Read the model definition and answer for the solid it produces. Units are mm, in the model's axes. Coordinates: 2 decimals unless noted, no trailing zeros. Loops run counter-clockwise (first coordinate to the right, second up) from the corner with the lowest first, then second, coordinate; pieces in that order, holes last. Notation, with made-up numbers: (73.25, -35) -> (118.25, -35) arc R6 ccw to (118.25, -25) -> close; hole circle Ø6 at (-28.75, -19). An arc over 180 degrees is marked (long way). Answer as a JSON object with one key per item and string values. Group by question number.
1) Section C-C, the plane z = 4.25 is taken. Give the vertices of the cut face in (x, y).
2) Consider probe 1 along Y at (x, z) = (0, 18.75); probe 2 along X at (y, z) = (3.5, 1.5); probe 3 along Y at (x, z) = (-1, 21.5). Determine where each line is inside the solid, lowest interval first. Write a range as [from, to].
3) Flat-ended cylindrical pins translate along their axes: P1, Ø1.5, axis at x = 1, z = 9.5, coming from the -Y side; P2, Ø1.5, axis at x = -4, z = 20.5, coming from the -Y side; P3, Ø1, axis at y = -2, z = 4.5, coming from the +X side. Find the tip coordinate at first contact, or state that the pin passes through.
4) Section A-A, the plane x = 0 is taken. Give the vertices of the cut face in (y, z), plus the area to 3 significant figures.
5) Determine the mould class of faces 1 (the face through (-0.867, -3.905, 12.161)), 2 (the face through (-7.493, -0.33, 11.839)), 3 (the face through (5, 0, 0)) for opening direction X: released by +X, released by -X, zero draft, split by the parting line, or undercut.
Autodesk Inventor part; units mm, degrees
ref_plane "YZ Plane" through (0, 0, 0) normal (1, 0, 0) x (0, 1, 0)
ref_plane "XZ Plane" through (0, 0, 0) normal (0, 1, 0) x (-1, 0, 0)
ref_plane "XY Plane" through (0, 0, 0) normal (0, 0, 1) x (1, 0, 0)
sketch "Sketch1" plane through (0, 0, 0) normal (0, 0, 1) x (1, 0, 0)
  circle A0 centre (0, 0) radius 7.5
  dimension "d0" = 15
extrude "Extrusion1" add sketch "Sketch1" along normal blind 24
sketch "Sketch2" plane through (0, 0, 24) normal (0, 0, 1) x (1, 0, 0)
  circle A0 centre (0, 0) radius 4
  dimension "d3" = 8
extrude "Extrusion2" cut sketch "Sketch2" against normal through all
chamfer "Chamfer1" distance 0.508 angle 45 4 edges at (-7.5, 0, 24) (-4, 0, 24) (-7.5, 0, 0) (-4, 0, 0)
properties part number "lm8uu rough model"
Determined:
{
 "1": {"outline": "circle Ø15 at (0, 0); hole circle Ø8 at (0, 0)"},
 "2": {"probe 1": "[-7.5, -4], [4, 7.5]", "probe 2": "[-6.63, -1.94], [1.94, 6.63]", "probe 3": "[-7.43, -3.87], [3.87, 7.43]"},
 "3": {"P1": "y = -7.5", "P2": "y = -6.76", "P3": "x = 7.35"},
 "4": {"outline": "(-7.5, 0.51) -> (-6.99, 0) -> (-4.51, 0) -> (-4, 0.51) -> (-4, 23.49) -> (-4.51, 24) -> (-6.99, 24) -> (-7.5, 23.49) -> close; (4, 0.51) -> (4.51, 0) -> (6.99, 0) -> (7.5, 0.51) -> (7.5, 23.49) -> (6.99, 24) -> (4.51, 24) -> (4, 23.49) -> close", "area": "167 mm²"},
 "5": {"face 1": "undercut", "face 2": "split by the parting line", "face 3": "zero draft"}
}
